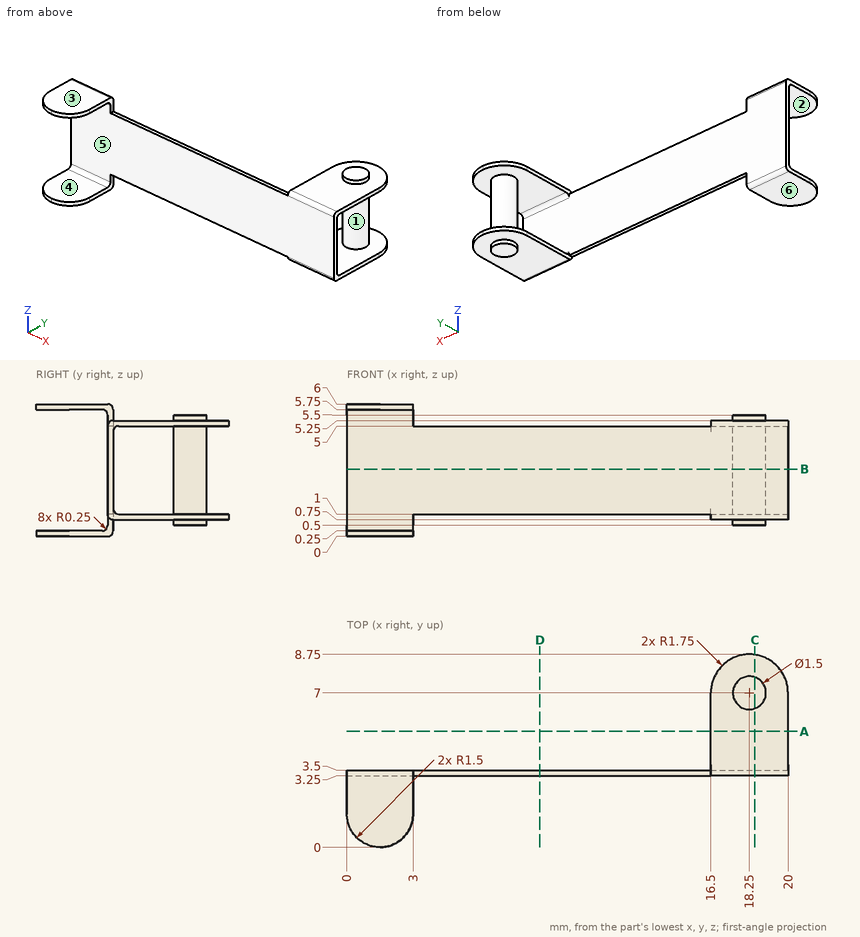
Here's the drawing with two shaded views (mm, measured from the low corner). I have some questions. A direction names the side the tool comes from. Coordinates: 2 decimals unless noted, no trailing zeros. Order: outer loops, then holes, each group sorted by start corner. A loop starts at its lowest first (then second) coordinate and runs counter-clockwise, first axis right, second up. Notation, with made-up numbers: (44.5, 25.25) -> (86.5, 25.25) arc R18 cw to (86.5, 42.25) -> close; hole circle Ø5 at (53, 35.25). An arc over 180 degrees is marked (long way). Write each question's results on one line, items separated by ' | '.
Item 1: Which directions (+Z, -Z, +X, -X, +Y, -Y) give clear straight access to the entire face, cutting with the end or side of a thin tool? Please do the marked faces 1 and 2.
Results are:
face 1: none | face 2: +X, -X, -Y
Item 2: If I drill on line 1 along Z through (x, y) = (18.25, 8.25); line 2 along Y through (x, z) = (16, 3.45); line 3 along X through (y, z) = (5.75, 5.2), over which ranges is the centre line in solid material (lowest first)?
Results are:
line 1: 0.75 to 1, 5 to 5.25 | line 2: 3.25 to 3.5 | line 3: 16.5 to 20
Item 3: I want a section at A-A, the plane y = 5.25. Write out the boundary of the cut face in (x, z), then the cut area to 3 significant figures.
Results are:
outline: (16.5, 0.75) -> (20, 0.75) -> (20, 1) -> (16.5, 1) -> close; (16.5, 5) -> (20, 5) -> (20, 5.25) -> (16.5, 5.25) -> close | area: 1.75 mm²
Item 4: I want a section at C-C, the plane x = 18.5. Write out the boundary of the cut face in (y, z), then the cut area to 3 significant figures.
Results are:
outline: (3.25, 1) arc R0.25 ccw to (3.5, 0.75) -> (6.29, 0.75) -> (6.29, 0.5) -> (7.71, 0.5) -> (7.71, 0.75) -> (8.73, 0.75) -> (8.73, 1) -> (7.71, 1) -> (7.71, 5) -> (8.73, 5) -> (8.73, 5.25) -> (7.71, 5.25) -> (7.71, 5.5) -> (6.29, 5.5) -> (6.29, 5.25) -> (3.5, 5.25) arc R0.25 ccw to (3.25, 5) -> close; hole (3.5, 1.25) arc R0.25 ccw to (3.75, 1) -> (6.29, 1) -> (6.29, 5) -> (3.75, 5) arc R0.25 ccw to (3.5, 4.75) -> close | area: 10.1 mm²
Item 5: I'm going to push flat-ended pins straight in: pin 1 Ø3 at (x, z) = (5, 2.5) entering from +Y; pin 2 Ø1 at (x, y) = (18, 7.5) entering from -Z; pin 3 Ø1 at (x, z) = (7, 2) entering from -Y. Where does each tip first touch, or does it pass through?
Results are:
pin 1: y = 3.5 | pin 2: z = 0.5 | pin 3: y = 3.25
Item 6: I want a section at B-B, the plane z = 3.05. Write out the boundary of the cut face in (x, y).
Results are:
outline: (0, 3.25) -> (20, 3.25) -> (20, 3.5) -> (0, 3.5) -> close; circle Ø1.5 at (18.25, 7)
Item 7: If we mould it in two halves opening along Z, with no side actions, what happens to the marked faces 3, 4, 5 and 6? For each: +Z half, -Z half, draft (parallel to the pull), parting line (faces both ways), or undercut.
Results are:
face 3: +Z half | face 4: undercut | face 5: undercut | face 6: -Z half
Item 8: I want a section at D-D, the plane x = 8.75. Write out the boundary of the cut face in (y, z).
Results are:
outline: (3.25, 1) -> (3.5, 1) -> (3.5, 5) -> (3.25, 5) -> close
